The listing builds one solid part. Answer for the finished solid, in the listing's coordinates (mm). Give positions to 0.01 mm unless a question says otherwise; leave off trailing zeros. Order: outer loops, then holes, each group sorted by start corner. A loop starts at its lowest first (then second) coordinate and runs counter-clockwise, first axis right, second up.
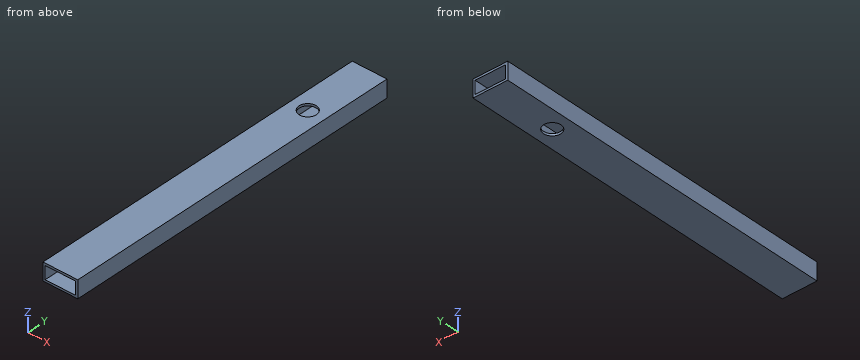
Autodesk Inventor part; units mm, degrees
ref_plane "YZ Plane" through (0, 0, 0) normal (1, 0, 0) x (0, 1, 0)
ref_plane "XZ Plane" through (0, 0, 0) normal (0, 1, 0) x (-1, 0, 0)
ref_plane "XY Plane" through (0, 0, 0) normal (0, 0, 1) x (1, 0, 0)
sketch "Sketch1" plane through (0, 0, 0) normal (0, 0, 1) x (1, 0, 0)
  line L0 (-25.4, -254) -> (25.4, -254)
  line L1 (25.4, -254) -> (25.4, 254)
  line L2 (25.4, 254) -> (-25.4, 254)
  line L3 (-25.4, 254) -> (-25.4, -254)
  line L4 (-25.4, -254) -> (25.4, 254) construction
  line L5 (25.4, -254) -> (-25.4, 254) construction
  point P0 (0, 0)
  dimension "d0" = 50.8
  dimension "d1" = 508
extrude "Extrusion1" add sketch "Sketch1" along normal mid plane 25.4
sketch "Sketch2" plane through (0, 0, 0) normal (0, 1, 0) x (-1, 0, 0)
  line L0 (-22.225, 9.525) -> (-22.225, -9.525)
  line L1 (-22.225, -9.525) -> (22.225, -9.525)
  line L2 (22.225, -9.525) -> (22.225, 9.525)
  line L3 (22.225, 9.525) -> (-22.225, 9.525)
  line L4 (-22.225, 9.525) -> (22.225, -9.525) construction
  line L5 (-22.225, -9.525) -> (22.225, 9.525) construction
  line L6 (25.4, -12.7) -> (25.4, 12.7)
  line L7 (25.4, 12.7) -> (-25.4, 12.7)
  point P0 (0, 0)
  dimension "d4" = 3.175
  dimension "d5" = 3.175
extrude "Extrusion2" cut sketch "Sketch2" along normal through all both and the other way through all
sketch "Sketch3" plane through (0, 0, 12.7) normal (0, 0, 1) x (1, 0, 0)
  line L0 (-22.225, 254) -> (22.225, 254) construction
  line L1 (0, 254) -> (0, -254) construction
  line L2 (22.225, -254) -> (-22.225, -254) construction
  point P0 (0, 0)
  point P1 (0, 152.4)
  dimension "d8" = 101.6
hole "Hole1" at (0, 152.4, 12.7) direction (0, 0, -1) diameter 25.4 end through all
equation "\"d0\" = width"
equation "\"d1\" = height"
equation "\"d2\" = depth"
equation "\"d4\" = wallThickness"
equation "\"d5\" = wallThickness"
equation "\"depth\" = 25.4"
equation "\"width\" = 50.8"
equation "\"height\" = 508"
equation "\"wallThickness\" = 3.175"
equation "\"distanceFromTopForOneInch\" = 101.6"
properties part number "sideExtrusion" material "Aluminum 6061"
1) Find section B-B (z = 4.5). Write down the section's boundary in (x, y) (3 decimals), then the cut area to 3 significant figures.
Geometry says:
outline: (-25.4, -254) - (-22.225, -254) - (-22.225, 254) - (-25.4, 254) - close; (22.225, -254) - (25.4, -254) - (25.4, 254) - (22.225, 254) - close
area: 3,230 mm2
2) Find section D-D (x = 0). Write down the section's boundary in (y, z) (3 decimals), then the cut area to 3 significant figures.
Geometry says:
outline: (-254, -12.7) - (139.7, -12.7) - (139.7, -9.525) - (-254, -9.525) - close; (-254, 9.525) - (139.7, 9.525) - (139.7, 12.7) - (-254, 12.7) - close; (165.1, -12.7) - (254, -12.7) - (254, -9.525) - (165.1, -9.525) - close; (165.1, 9.525) - (254, 9.525) - (254, 12.7) - (165.1, 12.7) - close
area: 3,060 mm2
3) Find section A-A (y = 152.4). Write down the section's boundary in (x, z) (3 decimals).
Geometry says:
outline: (-25.4, -12.7) - (-12.7, -12.7) - (-12.7, -9.525) - (-22.225, -9.525) - (-22.225, 9.525) - (-12.7, 9.525) - (-12.7, 12.7) - (-25.4, 12.7) - close; (12.7, -12.7) - (25.4, -12.7) - (25.4, 12.7) - (12.7, 12.7) - (12.7, 9.525) - (22.225, 9.525) - (22.225, -9.525) - (12.7, -9.525) - close
4) Straight lines are drawn through the part: probe 1 along X at (y, z) = (-167, -3) (3 decimals); probe 2 along X at (y, z) = (152.4, -11.75); probe 3 along Z at (x, y) = (-1, -149) (3 decimals). For each, find the intervals that lie inside material, in ascending order.
Geometry says:
probe 1: x = -25.4 to -22.225, 22.225 to 25.4
probe 2: x = -25.4 to -12.7, 12.7 to 25.4
probe 3: z = -12.7 to -9.525, 9.525 to 12.7
5) Find section C-C (y = -198). Write down the section's boundary in (x, z) (3 decimals), then the cut area to 3 significant figures.
Geometry says:
outline: (-25.4, -12.7) - (25.4, -12.7) - (25.4, 12.7) - (-25.4, 12.7) - close; hole (-22.225, -9.525) - (22.225, -9.525) - (22.225, 9.525) - (-22.225, 9.525) - close
area: 444 mm2
6) Given P1, Ø3, axis at x = 20, z = 2.5, coming from the -Y side, flat-ended and moving along its own axis, determine where the tip first touches the part or whether it passes through.
Geometry says:
P1: passes through
